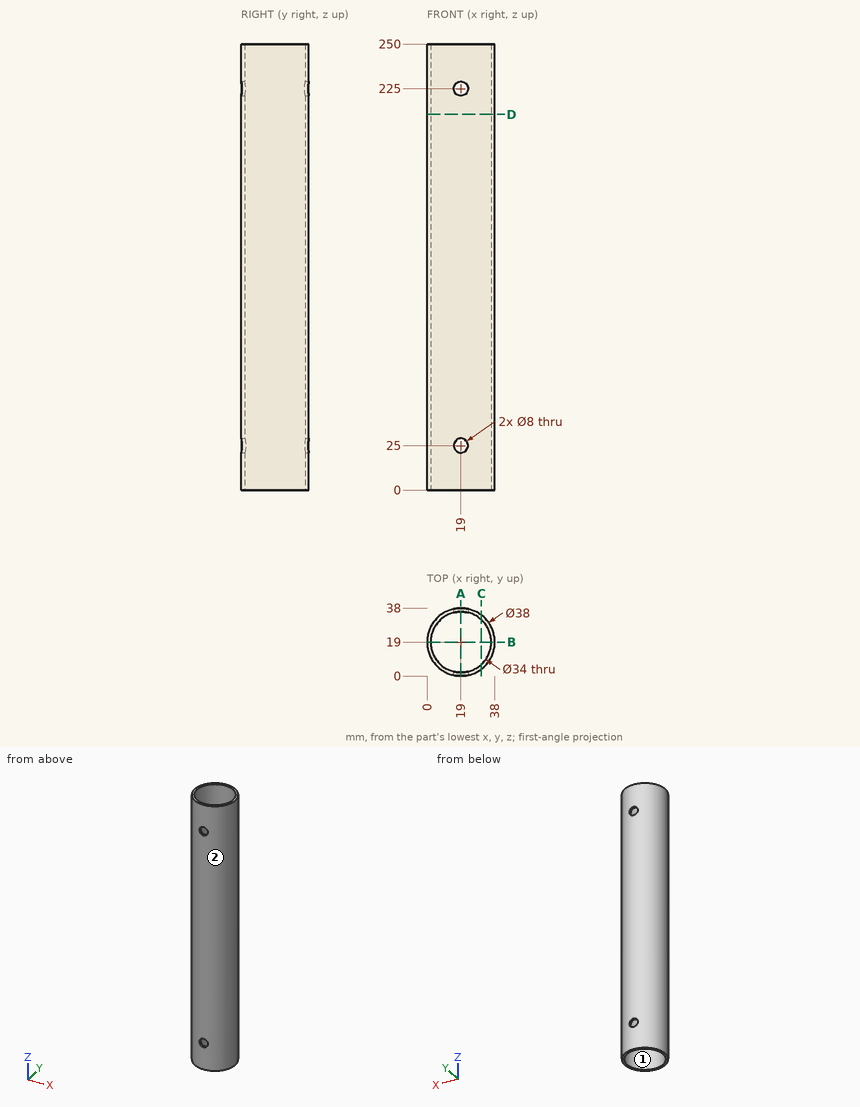
Answer from the drawing. Dimensions are ordinates in mm from the lowest x, y and z of the part. Give positions to 0.01 mm unless a question says otherwise; leave off trailing zeros. Order: outer loops, then holes, each group sorted by start corner. A loop starts at its lowest first (then second) coordinate and runs counter-clockwise, first axis right, second up. Notation, with made-up numbers: (81, -8.5) - (116, -8.5) arc R21 ccw to (116, 27.5) - close; hole circle Ø6 at (-35, 80.25). An arc over 180 degrees is marked (long way). One line per item, written item: value. Start each with the question number.
1. Section D-D, the plane z = 210.5 is taken. Write down the section's boundary in (x, y).
2. Section C-C, the plane x = 30.5 is taken. Write down the section's boundary in (y, z).
3. Section A-A, the plane x = 19 is taken. Write down the section's boundary in (y, z), then the cut area to 3 significant figures.
4. Consider line 1 (Z direction, x = 19, y = 37); line 2 (Y direction, x = 19, z = 72.5); line 3 (X direction, y = 19.5, z = 164). Determine where each line is inside the solid, lowest interval first.
5. Section B-B, the plane y = 19 is taken. Write down the section's boundary in (x, z).
6. Each of these flat-tipped pins is pushed along its axis until it touches: pin 1 Ø7 at (x, z) = (19, 25) entering from -Y (3 decimals); pin 2 Ø4 at (x, z) = (13.5, 220.5) entering from +Y; pin 3 Ø5 at (x, z) = (33.5, 126.5) entering from -Y; pin 4 Ø5 at (y, z) = (10.5, 65) entering from +X. Where does it stop, or does it pass through?
7. For a pull along X with two mould halves and no side action, classify the marked faces 1 and 2 as released by +X, released by -X, zero draft, split by the parting line, or undercut.
Filled sheet:
1. outline: circle Ø38 at (19, 19); hole circle Ø34 at (19, 19)
2. outline: (3.88, 0) - (6.48, 0) - (6.48, 250) - (3.88, 250) - close; (31.52, 0) - (34.12, 0) - (34.12, 250) - (31.52, 250) - close
3. outline: (0, 0) - (2, 0) - (2, 21) - (0, 21) - close; (0, 29) - (2, 29) - (2, 221) - (0, 221) - close; (0, 229) - (2, 229) - (2, 250) - (0, 250) - close; (36, 0) - (38, 0) - (38, 21) - (36, 21) - close; (36, 29) - (38, 29) - (38, 221) - (36, 221) - close; (36, 229) - (38, 229) - (38, 250) - (36, 250) - close
3. area: 936 mm²
4. line 1: 0 to 21, 29 to 221, 229 to 250
4. line 2: 0 to 2, 36 to 38
4. line 3: 0.01 to 2.01, 35.99 to 37.99
5. outline: (0, 0) - (2, 0) - (2, 250) - (0, 250) - close; (36, 0) - (38, 0) - (38, 250) - (36, 250) - close
6. pin 1: through
6. pin 2: y = 37.67
6. pin 3: y = 4.27
6. pin 4: x = 37.03
7. face 1: undercut
7. face 2: split by the parting line
